Part model, mm, in its own coordinate system. Face numbers are marked on the shaded views. A direction names the side the tool comes from. Give positions to 0.01 mm unless a question says otherwise; leave off trailing zeros. Order: outer loops, then holes, each group sorted by start corner. A loop starts at its lowest first (then second) coordinate and runs counter-clockwise, first axis right, second up. Notation, with made-up numbers: M -26,13.5 L -1,13.5 A21 cw -1,18.5 Z; hole C -34.5,24 d3. An arc over 180 degrees is marked long. Return JSON: item names as keys, results as strings.
from build123d import *

# Parameters (mm, degrees)
F0_W          = 81.28
F0_H          = 31.75
F1_DEPTH      = 19.05
F3_DEPTH      = 19.304
F3_DEPTH_BACK = 19.05
F4_DEPTH      = 19.05


with BuildPart() as f1:
    # F0 (on Top) → F1 (new body)
    with BuildSketch(Plane.XY):
        Rectangle(F0_W, F0_H)
    extrude(amount=F1_DEPTH)

    # F2 (on Top) → F3 (cut, two sides)
    with BuildSketch(Plane.XY) as f3_sk:
        with BuildLine():
            ThreePointArc((-16.953665, 6.985), (-23.940335, 0.000835), (-16.955335, -6.985))
            Line((-16.955335, -6.985), (16.953665, -6.985))
            ThreePointArc((16.953665, -6.985), (23.938665, -0.000835), (16.955335, 6.985))
            Line((16.955335, 6.985), (-16.953665, 6.985))
        make_face()
    extrude(amount=F3_DEPTH, mode=Mode.SUBTRACT)
    extrude(f3_sk.sketch, amount=-F3_DEPTH_BACK, mode=Mode.SUBTRACT)

    # F0 (on Top) → F4 (join)
    with BuildSketch(Plane.XY):
        Polygon((-40.64, -15.875), (-40.64, 15.875), (-59.514749, 4.778779), (-59.853135, -5.375585), align=None)
    extrude(amount=F4_DEPTH)


solid = f1.part
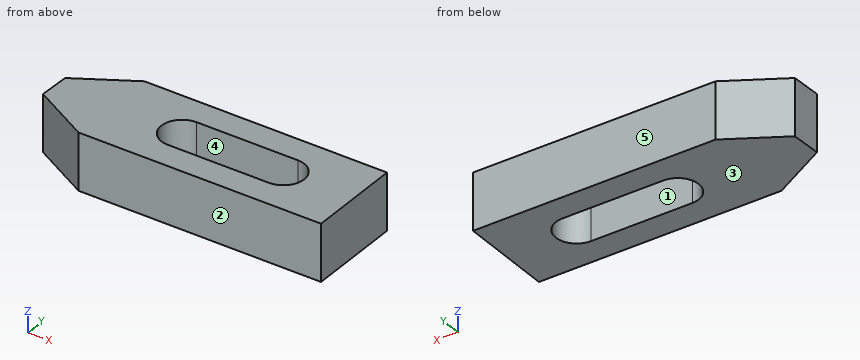
Q1. Pin check, flat tip, straight feed: pin 1 (3 mm diameter, centred on y = 4.5, z = 9, fed in from -X). Stop position of the tip, or through.
Established:
{"pin 1": "stops at x = -59.57"}
Q2. Band-saw the part on D-D (y = 8). Give the cut face in (x, z).
Established:
{"outline": "M -54.04,0 L 40.64,0 L 40.64,19.05 L -54.04,19.05 Z"}
Q3. Band-saw the part on C-C (y = 0). Give the cut face in (x, z).
Established:
{"outline": "M -59.67,0 L -23.94,0 L -23.94,19.05 L -59.67,19.05 Z; M 23.94,0 L 40.64,0 L 40.64,19.05 L 23.94,19.05 Z"}
Q4. Band-saw the part on A-A (x = -11.5). Give the cut face in (y, z) (3 decimals), then the cut area to 3 significant figures.
Established:
{"outline": "M -15.875,0 L -6.985,0 L -6.985,19.05 L -15.875,19.05 Z; M 6.985,0 L 15.875,0 L 15.875,19.05 L 6.985,19.05 Z", "area": "339 mm²"}
Q5. Band-saw the part on B-B (z = 8). Give the cut face in (x, y) (3 decimals), then the cut area to 3 significant figures.
Established:
{"outline": "M -59.853,-5.376 L -40.64,-15.875 L 40.64,-15.875 L 40.64,15.875 L -40.64,15.875 L -59.515,4.779 Z; hole M -16.955,-6.985 L 16.954,-6.985 A6.985 ccw 16.955,6.985 L -16.954,6.985 A6.985 ccw Z", "area": "2,350 mm²"}
Q6. Two-plate mould, pull along Y, no slides. Class the marked faces 1, 2 and 3: +Y half, -Y half, draft (parallel to the pull), parting line (faces both ways), or undercut.
Established:
{"face 1": "undercut", "face 2": "-Y half", "face 3": "draft"}
Q7. 3-axis set-ups, long thin cutter, end or side, ignore diameter. For the marked faces 4 and 5: which of +Z, -Z, +X, -X, +Y, -Y reach the whole face in a straight line?
Established:
{"face 4": "+Z, -Z", "face 5": "+Z, -Z, +X, -X, +Y"}
Q8. Probe line 1 along Y through (x, z) = (1.5, 16.75) (3 decimals); line 2 along X through (y, z) = (4.5, 2); line 3 along X through (y, z) = (-5.5, 9). List the from-to ranges inside material, lowest first.
Established:
{"line 1": "y = -15.875 to -6.985, 6.985 to 15.875", "line 2": "x = -59.52 to -22.3, 22.3 to 40.64", "line 3": "x = -59.63 to -21.26, 21.26 to 40.64"}
